```python
from build123d import *

# Parameters (mm, degrees)
SKETCH1_R             = 7.5
BOSS_EXTRUDE1_DEPTH   = 2.5
SKETCH2_R             = 9
BOSS_EXTRUDE2_DEPTH   = 0.9
SKETCH3_R             = 10
BOSS_EXTRUDE3_DEPTH   = 22
SKETCH5_R             = 2.7
CUT_EXTRUDE1_DEPTH    = 5.5
CUT_EXTRUDE2_DEPTH    = 19
SKETCH7_R             = 2.7
CUT_EXTRUDE3_DEPTH    = 30.071635661
CIRPATTERN1_START     = 2.951270805
CIRPATTERN1_OUTLINE_R = 2.7
CIRPATTERN1_DEPTH     = 7.048729295
CHAMFER1_SIZE         = 0.3


# Read off the part's stored shape, not the designer's step: CirPattern1
with BuildPart() as part:
    # Sketch1 → Boss-Extrude1 (new body)
    with BuildSketch(Plane(origin=(0, 0, 0), x_dir=(1, 0, 0), z_dir=(0, 1, 0))):
        with Locations(Location((0, 0, 0), (0, 0, 270))):
            Circle(SKETCH1_R)
    extrude(amount=BOSS_EXTRUDE1_DEPTH)

    # Sketch2 → Boss-Extrude2 (add)
    with BuildSketch(Plane(origin=(0, 2.5, 0), x_dir=(1, 0, 0), z_dir=(0, 1, 0))):
        with Locations(Location((0, 0, 0), (0, 0, 270))):
            Circle(SKETCH2_R)
    extrude(amount=BOSS_EXTRUDE2_DEPTH)

    # Sketch3 → Boss-Extrude3 (add)
    with BuildSketch(Plane(origin=(0, 3.4, 0), x_dir=(1, 0, 0), z_dir=(0, 1, 0))):
        with Locations(Location((0, 0, 0), (0, 0, 270))):
            Circle(SKETCH3_R)
    extrude(amount=BOSS_EXTRUDE3_DEPTH)

    # Sketch5 → Cut-Extrude1 (cut)
    with BuildSketch(Plane.XZ):
        with Locations(Location((3.6, 0, 0), (0, 0, 270))):
            Circle(SKETCH5_R)
        with Locations(Location((-3.6, 0, 0), (0, 0, 270))):
            Circle(SKETCH5_R)
    extrude(amount=-CUT_EXTRUDE1_DEPTH, mode=Mode.SUBTRACT)

    # Sketch6 → Cut-Extrude2 (cut)
    with BuildSketch(Plane(origin=(0, 25.4, 0), x_dir=(1, 0, 0), z_dir=(0, 1, 0))):
        with BuildLine():
            Line((-1.936491673, 3.5), (1.936491673, 3.5))
            ThreePointArc((1.936491673, 3.5), (0, -4), (-1.936491673, 3.5))
        make_face()
    extrude(amount=-CUT_EXTRUDE2_DEPTH, mode=Mode.SUBTRACT)

    # Sketch7 → Cut-Extrude3 (cut, through all)
    with BuildSketch(Plane.XY):
        with Locations(Location((0, 18.4, 0), (0, 0, 315.82536203))):
            Circle(SKETCH7_R)
    extrude(amount=-CUT_EXTRUDE3_DEPTH, mode=Mode.SUBTRACT)

    # CirPattern1 outline → CirPattern1 (cut)
    with BuildSketch(Plane(origin=(0, 0, 0), x_dir=(0.7071067811865509, 0, -0.707106781186544), z_dir=(0.707106781186544, 0, 0.707106781186551)).offset(CIRPATTERN1_START)):
        with Locations((0, 18.4)):
            Circle(CIRPATTERN1_OUTLINE_R)
    extrude(amount=CIRPATTERN1_DEPTH, mode=Mode.SUBTRACT)

    # Chamfer1
    chamfer1_edges = [part.edges().sort_by_distance(p)[0] for p in [
        (0, 0, -7.5),
    ]]
    chamfer(chamfer1_edges, length=CHAMFER1_SIZE)


solid = part.part
```
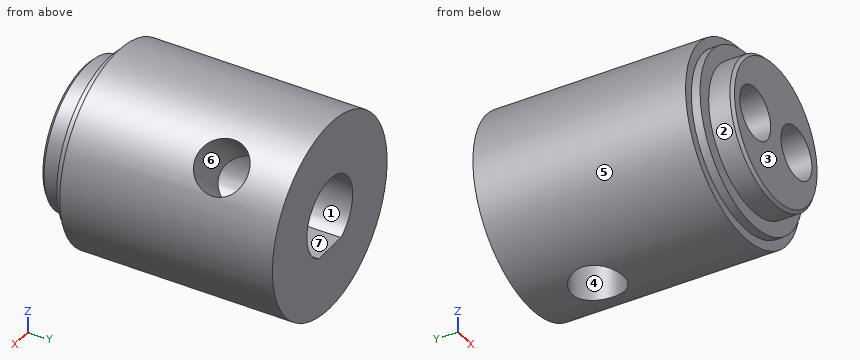
For this review, take the finished solid that the model builds, in its own axes (mm). Face numbers are marked on the shaded views. A direction names the side the tool comes from. Coordinates: 2 decimals unless noted, no trailing zeros. Write each loop counter-clockwise with the first axis right and the second up, starting at its lowest first coordinate (ties: lowest second). Pieces come first, ordered by that corner, then holes.
(1) Add section A-A on y = 3.75. Give the boundary of the cut face in (x, z), then the cut area to 3 significant figures.
(2) Tool access review of the marked faces 1, 2 and 3: name each direction out of +Z, -Z, +X, -X, +Y, -Y from which nothing blocks a thin tool from reaching the whole face with its end or side.
(3) The part is to be moulded in two halves that separate along Z. For the marked faces 4, 5, 6 and 7, say which applies: +Z half, -Z half, draft (parallel to the pull), parting line (faces both ways), or undercut.
(4) Add section C-C on y = 8.5. Give the boundary of the cut face in (x, z), then the cut area to 3 significant figures.
(5) Add section B-B on y = 17.25. Give the boundary of the cut face in (x, z), then the cut area to 3 significant figures.
(6) Wall thickness on probe 1 along X at (y, z) = (4.45, 0); probe 2 along X at (y, z) = (1.3, 0); probe 3 along Z at (x, y) = (0, 14.5): over which ranges is each line inside the solid? List them lowest first.
(7) For pin 1 Ø3 at (x, z) = (-3.6, 0) entering from -Y; pin 2 Ø5 at (x, y) = (-7.5, 16.5) entering from +Z; pin 3 Ø5 at (x, z) = (3.6, 0) entering from +Y; pin 4 Ø6 at (x, y) = (-5.5, 22) entering from +Z, all flat-tipped, find the tip position at first contact; note any pin that passes through.
Answer sheet:
1. outline: circle Ø20 at (0, 0); hole circle Ø5.4 at (-3.6, 0); hole circle Ø5.4 at (3.6, 0)
1. area: 268 mm2
2. face 1: +Y
2. face 2: -Y
2. face 3: +Z, -Z, +X, -X, -Y
3. face 4: draft
3. face 5: parting line
3. face 6: undercut
3. face 7: undercut
4. outline: circle Ø20 at (0, 0); hole (-1.94, -3.5) - (1.94, -3.5) arc R4 ccw (long way) to start
4. area: 265 mm2
5. outline: (-2.44, -9.7) - (-2.44, -3.17) arc R4 cw to (0.51, 3.97) - (5.13, 8.58) arc R10 ccw (long way) to start; (2.44, -9.7) arc R10 ccw to (8.58, 5.13) - (3.97, 0.51) arc R4 cw to (2.44, -3.17) - close
5. area: 204 mm2
6. probe 1: x = -10 to -6.3, -0.9 to 0.9, 6.3 to 10
6. probe 2: x = -7.5 to -6.3, -0.9 to 0.9, 6.3 to 7.5
6. probe 3: z = -10 to -3.5, 4 to 10
7. pin 1: stops at y = 5.5
7. pin 2: stops at z = 8.66
7. pin 3: stops at y = 25.4
7. pin 4: stops at z = 9.68
